The listing builds one solid part. Answer for the finished solid, in the listing's coordinates (mm). A direction names the side the tool comes from. Give positions to 0.01 mm unless a question says otherwise; leave off trailing zeros. Order: outer loops, then holes, each group sorted by start corner. A loop starts at its lowest first (then second) coordinate and runs counter-clockwise, first axis right, second up.
```python
from build123d import *

# Parameters (mm, degrees)
F0_R     = 2.75
F1_DEPTH = 4
F2_R     = 12.5
F3_DEPTH = 4.5
F4_R     = 5.5
F4_R_2   = 4
F5_DEPTH = 13


with BuildPart() as f1:
    # F0 (on Top) → F1 (new body)
    with BuildSketch(Plane.XY):
        with BuildLine():
            Line((-20.691781, -5.205786), (-5.732877, -12.22228))
            ThreePointArc((-5.732877, -12.22228), (0, -13.5), (5.732877, -12.22228))
            Line((5.732877, -12.22228), (20.691781, -5.205786))
            ThreePointArc((20.691781, -5.205786), (24, 0), (20.691781, 5.205786))
            Line((20.691781, 5.205786), (5.732877, 12.22228))
            ThreePointArc((5.732877, 12.22228), (0, 13.5), (-5.732877, 12.22228))
            Line((-5.732877, 12.22228), (-20.691781, 5.205786))
            ThreePointArc((-20.691781, 5.205786), (-24, 0), (-20.691781, -5.205786))
        make_face()
        with Locations((-18.25, 0)):
            Circle(F0_R, mode=Mode.SUBTRACT)
        with Locations((18.25, 0)):
            Circle(F0_R, mode=Mode.SUBTRACT)
    extrude(amount=F1_DEPTH)

    # F2 (on face) → F3 (join)
    with BuildSketch(Plane.XY.offset(4)):
        Circle(F2_R)
    extrude(amount=F3_DEPTH)

    # F4 (on face) → F5 (join)
    with BuildSketch(Plane(origin=(0, 0, 0), x_dir=(1, 0, 0), z_dir=(0, 0, -1))):
        Circle(F4_R)
        Circle(F4_R_2, mode=Mode.SUBTRACT)
    extrude(amount=-F5_DEPTH)


solid = f1.part
```
1) Find section C-C (x = 0). Write down the section's boundary in (y, z), then the cut area to 3 significant figures.
Geometry says:
outline: (-13.5, 0) - (13.5, 0) - (13.5, 4) - (12.5, 4) - (12.5, 8.5) - (5.5, 8.5) - (5.5, 13) - (4, 13) - (4, 8.5) - (-4, 8.5) - (-4, 13) - (-5.5, 13) - (-5.5, 8.5) - (-12.5, 8.5) - (-12.5, 4) - (-13.5, 4) - close
area: 234 mm2
2) Find section D-D (z = 11.5). Write down the section's boundary in (x, y).
Geometry says:
outline: circle Ø11 at (0, 0); hole circle Ø8 at (0, 0)
3) Given P1, Ø1, axis at x = 3, y = 6, coming from the +Z side; P2, Ø6.5, axis at x = 18.25, y = 0, coming from the +Z side; P3, Ø4.5, axis at x = -18.25, y = 0, coming from the +Z side; P4, Ø1.5, axis at y = 4.5, z = 7, coming from the -X side, each flat-ended and moving along its own axis, determine where each tip first touches the part or whether it passes through.
Geometry says:
P1: stops at z = 8.5
P2: stops at z = 4
P3: passes through
P4: stops at x = -11.92
4) A tool of negligible diameter and unlimited length cuts with its end or side. For faces 1 (the cylindrical face through (11.923, 3.755, 6.219)), 2 (the cylindrical face through (-0.1, -13.5, 2)), from which of +Z, -Z, +X, -X, +Y, -Y can it reach the whole face along a straight path? Write none if from no direction.
Geometry says:
face 1: +Z
face 2: +Z, -Z, -Y
5) For a pull along X with two mould halves and no side action, classify faces 3 (the cylindrical face through (16.068, -1.673, 1.972)), 4 (the flat face through (0, 0, 8.5)), 5 (the cylindrical face through (24, 0, 2)), 6 (the cylindrical face through (0.1, 13.5, 2)) as +X half, -X half, draft (parallel to the pull), parting line (faces both ways), or undercut.
Geometry says:
face 3: undercut
face 4: undercut
face 5: +X half
face 6: parting line
6) Find section A-A (y = 0). Write down the section's boundary in (x, z).
Geometry says:
outline: (-24, 0) - (-21, 0) - (-21, 4) - (-24, 4) - close; (-15.5, 0) - (15.5, 0) - (15.5, 4) - (12.5, 4) - (12.5, 8.5) - (5.5, 8.5) - (5.5, 13) - (4, 13) - (4, 8.5) - (-4, 8.5) - (-4, 13) - (-5.5, 13) - (-5.5, 8.5) - (-12.5, 8.5) - (-12.5, 4) - (-15.5, 4) - close; (21, 0) - (24, 0) - (24, 4) - (21, 4) - close
7) Find section B-B (z = 3.25). Write down the section's boundary in (x, y).
Geometry says:
outline: (-20.69, -5.21) - (-5.73, -12.22) arc R13.5 ccw to (5.73, -12.22) - (20.69, -5.21) arc R5.75 ccw to (20.69, 5.21) - (5.73, 12.22) arc R13.5 ccw to (-5.73, 12.22) - (-20.69, 5.21) arc R5.75 ccw to start; hole circle Ø5.5 at (-18.25, 0); hole circle Ø5.5 at (18.25, 0)
8) Straight lines are drawn through the part: probe 1 along Y at (x, z) = (0, 11.05); probe 2 along Z at (x, y) = (-6, -7); probe 3 along Z at (x, y) = (-14, 5.5). For each, find the intervals that lie inside material, in ascending order.
Geometry says:
probe 1: y = -5.5 to -4, 4 to 5.5
probe 2: z = 0 to 8.5
probe 3: z = 0 to 4
